from build123d import *

# Parameters (mm, degrees)
BOSS_EXTRUDE1_DEPTH     = 157
FILLET1_R               = 5
CUT_EXTRUDE1_DEPTH      = 199.704151945
CUT_EXTRUDE1_DEPTH_BACK = 199.704151945
SKETCH2_W               = 141
SKETCH2_H               = 19.5
FILLET5_R               = 8
SKETCH4_W               = 1.487907189
SKETCH4_H               = 11
BOSS_EXTRUDE5_DEPTH     = 141


with BuildPart() as part:
    # Sketch1 → Boss-Extrude1 (new body)
    with BuildSketch(Plane.XY):
        with BuildLine():
            Line((-110.7, 13.791796068), (-110.7, 3))
            Line((-110.7, 3), (-4, 3))
            Line((-4, 3), (-4, 13.791796068))
            ThreePointArc((-4, 13.791796068), (-8.157630053, 17.170797072), (-8.708203932, 22.5))
            Line((-8.708203932, 22.5), (-6.582575695, 22.5))
            ThreePointArc((-6.582575695, 22.5), (-2, 15.5), (2.582575695, 22.5))
            Line((2.582575695, 22.5), (4.708203932, 22.5))
            ThreePointArc((4.708203932, 22.5), (4.157630053, 17.170797072), (0, 13.791796068))
            Line((0, 13.791796068), (0, 2))
            Line((0, 2), (0, 0))
            Line((0, 0), (-114.7, 0))
            Line((-114.7, 0), (-114.7, 2))
            Line((-114.7, 2), (-114.7, 13.791796068))
            ThreePointArc((-114.7, 13.791796068), (-118.857630053, 17.170797072), (-119.408203932, 22.5))
            Line((-119.408203932, 22.5), (-117.282575695, 22.5))
            ThreePointArc((-117.282575695, 22.5), (-112.7, 15.5), (-108.117424305, 22.5))
            Line((-108.117424305, 22.5), (-105.991796068, 22.5))
            ThreePointArc((-105.991796068, 22.5), (-106.542369947, 17.170797072), (-110.7, 13.791796068))
        make_face()
    extrude(amount=BOSS_EXTRUDE1_DEPTH)

    # Fillet1
    fillet1_edges = [part.edges().sort_by_distance(p)[0] for p in [
        (-110.7, 3, 78.5),
        (-4, 3, 78.5),
        (-4, 13.791796068, 78.5),
        (0, 13.791796068, 78.5),
        (0, 0, 78.5),
        (-114.7, 0, 78.5),
        (-114.7, 13.791796068, 78.5),
        (-110.7, 13.791796068, 78.5),
    ]]
    fillet(fillet1_edges, radius=FILLET1_R)

    # Sketch2 → Cut-Extrude1 (cut, two sides: drawn at the far end of the back side and taken through both)
    with BuildSketch(Plane.ZY.offset(114.7).offset(-CUT_EXTRUDE1_DEPTH_BACK)):
        with Locations((78.5, 12.75)):
            Rectangle(SKETCH2_W, SKETCH2_H)
    extrude(amount=CUT_EXTRUDE1_DEPTH + CUT_EXTRUDE1_DEPTH_BACK, mode=Mode.SUBTRACT)

    # Fillet5
    fillet5_edges = [part.edges().sort_by_distance(p)[0] for p in [
        (-4.708712153, 3, 8),
        (-4.708712153, 3, 149),
        (-109.991287847, 3, 149),
        (-109.991287847, 3, 8),
    ]]
    fillet(fillet5_edges, radius=FILLET5_R)

    # Sketch4 → Boss-Extrude5 (add)
    with BuildSketch(Plane.XY.offset(8)):
        with Locations((-113.538622101, 8.5)):
            Rectangle(SKETCH4_W, SKETCH4_H)
        with Locations((-1.1613779, 8.5)):
            Rectangle(SKETCH4_W, SKETCH4_H)
    extrude(amount=BOSS_EXTRUDE5_DEPTH)


solid = part.part
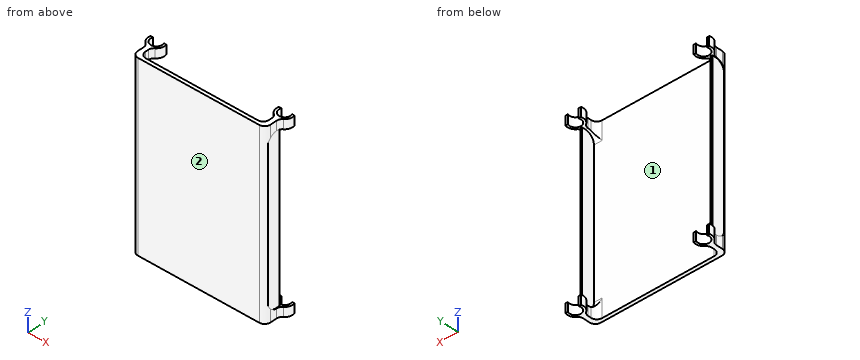
Source: CAD feature listing. Evaluate the final solid. Frame: model axes, mm. Face numbers are marked on the shaded views. Round coordinates to 2 decimals unless told otherwise and drop trailing zeros. Loops run counter-clockwise (first coordinate to the right, second up) from the corner with the lowest first, then second, coordinate; pieces in that order, holes last. Notation, with made-up numbers: (6, -26.5) - (10, -26.5) arc R34 cw to (10, 7.5) - close; hole circle Ø4 at (3, 40). An arc over 180 degrees is marked (long way). Write item = value, one per line. Start each with the question number.
Item 1: Section query A-A on y = 20.5. Count the separate pieces of the cut face and the enclosed holes in it, plus the area to 3 significant figures.
Item 2: Mould query, pull axis X, two halves, no side actions, for the marked faces 1 and 2. Classes: released by +X, released by -X, zero draft, split by the parting line, or undercut.
Item 3: Section query B-B on x = -80. Output: boundary loops of the cut face in (y, z).
Item 4: Material intervals for line 1 (X direction, y = 20.5, z = 155); line 2 (X direction, y = 9.25, z = 91.5); line 3 (X direction, y = 9, z = 151), sorted ascending.
Item 5: First-contact query: pin 1 Ø8 at (y, z) = (16, 90) entering from +X; pin 2 Ø3 at (y, z) = (8.5, 6.5) entering from +X; pin 3 Ø1 at (x, z) = (-84.5, 108.5) entering from +Y. Flat tips, straight axial feed; report the tip coordinate or a pass-through.
Results list:
q1.separate_pieces = 8
q1.enclosed_holes = 0
q1.area = 128 mm²
q2.face_1 = undercut
q2.face_2 = zero draft
q3.outline = (0, 0) - (3, 0) - (3, 157) - (0, 157) - close
q4.line_1 = -119.7 to -117.7, -107.7 to -105.7, -9 to -7, 3 to 5
q4.line_2 = -114.28 to -112.79, -1.91 to -0.42
q4.line_3 = -114.7 to -110.7, -4 to 0
q5.pin_1 = -0.42
q5.pin_2 = 0
q5.pin_3 = 3
